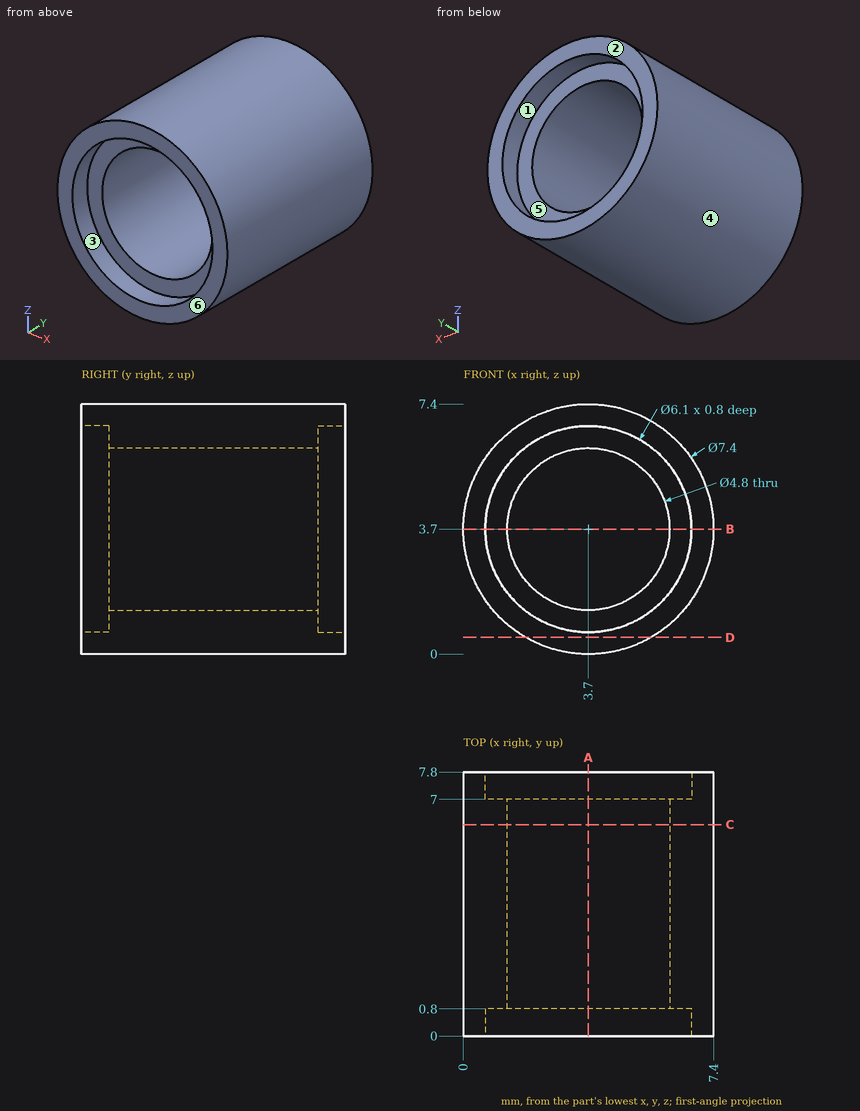
Can you work these out from the drawing? Everything is in mm from the part's minimum corner. A direction names the side the tool comes from. Coordinates: 2 decimals unless noted, no trailing zeros. Write each loop counter-clockwise with the first axis right and the second up, starting at its lowest first coordinate (ties: lowest second). Pieces come first, ordered by that corner, then holes. Notation, with made-up numbers: (-8.5, -20.75) - (35.5, -20.75) arc R33 ccw to (35.5, 18.25) - close; hole circle Ø2 at (-24.5, 68.25). An arc over 180 degrees is marked (long way). One line per item, written item: value.
1) Suppose I cut it at C-C on y = 6.25. Write out the boundary of the cut face in (x, z).
Model answer:
outline: circle Ø7.4 at (3.7, 3.7); hole circle Ø4.8 at (3.7, 3.7)
2) Suppose I cut it at A-A on x = 3.7. Write out the boundary of the cut face in (y, z), and give its area (3 significant figures).
Model answer:
outline: (0, 0) - (7.8, 0) - (7.8, 0.65) - (7, 0.65) - (7, 1.3) - (0.8, 1.3) - (0.8, 0.65) - (0, 0.65) - close; (0, 6.75) - (0.8, 6.75) - (0.8, 6.1) - (7, 6.1) - (7, 6.75) - (7.8, 6.75) - (7.8, 7.4) - (0, 7.4) - close
area: 18.2 mm²
3) I need wall thicknesses on line 1 along X through (y, z) = (3, 3.7); line 2 along Z through (x, y) = (3.7, 0.65). Which ranges of each line are inside material? Lowest first, please.
Model answer:
line 1: x = 0 to 1.3, 6.1 to 7.4
line 2: z = 0 to 0.65, 6.75 to 7.4
4) Suppose I cut it at B-B on z = 3.7. Write out the boundary of the cut face in (x, y), and give its area (3 significant figures).
Model answer:
outline: (0, 0) - (0.65, 0) - (0.65, 0.8) - (1.3, 0.8) - (1.3, 7) - (0.65, 7) - (0.65, 7.8) - (0, 7.8) - close; (6.1, 0.8) - (6.75, 0.8) - (6.75, 0) - (7.4, 0) - (7.4, 7.8) - (6.75, 7.8) - (6.75, 7) - (6.1, 7) - close
area: 18.2 mm²
5) On a 3-axis mill with a long thin cutter (end or side, diameter ignored), from which of +Z, -Z, +X, -X, +Y, -Y can I reach the whole of each face in a straight line? I mean the marked faces 1, 2 and 3. Say none if no direction works.
Model answer:
face 1: +Y
face 2: +Z, -Z, +X, -X, +Y
face 3: -Y
6) We'd pull the mould along X, two halves only. Please class the marked faces 4, 5 and 6: pulls with the +X half, pulls with the -X half, needs draft (parallel to the pull), parting line crosses it, or undercut.
Model answer:
face 4: parting line crosses it
face 5: undercut
face 6: needs draft
7) Suppose I cut it at D-D on z = 0.5. Write out the boundary of the cut face in (x, y).
Model answer:
outline: (1.84, 0) - (5.56, 0) - (5.56, 7.8) - (1.84, 7.8) - close
